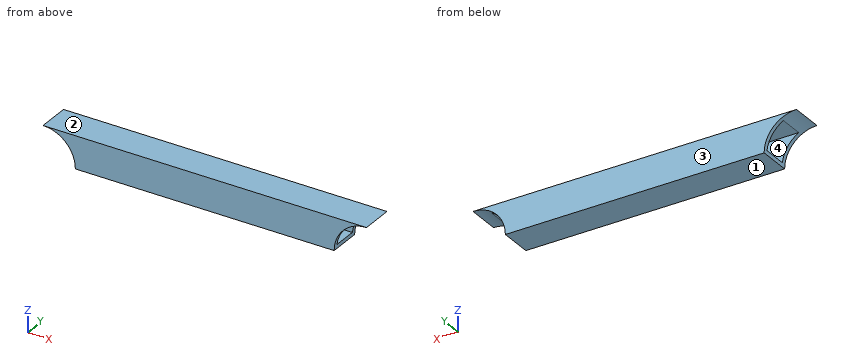
from build123d import *

# Parameters (mm, degrees)
BOSS_EXTRUDE1_DEPTH     = 25.4
CUT_EXTRUDE1_DEPTH      = 163.851117067
CUT_EXTRUDE1_DEPTH_BACK = 163.851117067
SKETCH2_W               = 19.05
SKETCH2_H               = 19.05


with BuildPart() as part:
    # Sketch1 → Boss-Extrude1 (new body)
    with BuildSketch(Plane(origin=(0, 0, 0), x_dir=(1, 0, 0), z_dir=(0, 1, 0))):
        with BuildLine():
            Line((-127, -98.723484187), (127, -98.723484187))
            ThreePointArc((127, -98.723484187), (109.039487758, -91.283996429), (101.6, -73.323484187))
            Line((101.6, -73.323484187), (-101.6, -73.323484187))
            ThreePointArc((-101.6, -73.323484187), (-109.039487758, -91.283996429), (-127, -98.723484187))
        make_face()
    extrude(amount=BOSS_EXTRUDE1_DEPTH)

    # Sketch2 → Cut-Extrude1 (cut, two sides: drawn at the far end of the back side and taken through both)
    with BuildSketch(Plane(origin=(0, 0, 0), x_dir=(0, 0, -1), z_dir=(1, 0, 0)).offset(-CUT_EXTRUDE1_DEPTH_BACK)):
        with Locations((-86.023484187, 12.7)):
            Rectangle(SKETCH2_W, SKETCH2_H)
    extrude(amount=CUT_EXTRUDE1_DEPTH + CUT_EXTRUDE1_DEPTH_BACK, mode=Mode.SUBTRACT)


solid = part.part
Model file for the job. Use its own axes, mm. Face numbers are marked on the shaded views. Round coordinates to 2 decimals unless told otherwise and drop trailing zeros. Order: outer loops, then holes, each group sorted by start corner. A loop starts at its lowest first (then second) coordinate and runs counter-clockwise, first axis right, second up.
(1) Drill centre lines: line 1 (Y direction, x = -57, z = 79.5) (3 decimals); line 2 (Z direction, x = 17, y = 13.25); line 3 (Z direction, x = -112, y = 5.5). Where is each one in solid material? Low to high.
(2) Band-saw the part on C-C (z = 83.5). List the corners of the cut face in (x, y) (3 decimals), then the cut area to 3 significant figures.
(3) Band-saw the part on B-B (x = 41). List the corners of the cut face in (y, z) (3 decimals), then the cut area to 3 significant figures.
(4) Band-saw the part on A-A (y = 8.5). List the corners of the cut face in (x, z).
(5) Pull direction Z, two halves, no side cores. Call the marked faces 1, 2, 3 and 4: released by +Z, released by -Z, zero draft, split by the parting line, or undercut.
(6) Pin check, flat tips, straight feed: pin 1 (10 mm diameter, centred on y = 19.5, z = 90, fed in from -X); pin 2 (5 mm diameter, centred on x = -88.5, z = 76.5, fed in from -Y); pin 3 (6 mm diameter, centred on y = 9, z = 86, fed in from -X). Stop position of each tip, or through.
Verdict:
1. line 1: y = 0 to 3.175, 22.225 to 25.4
1. line 2: z = 73.32 to 76.5, 95.55 to 98.72
1. line 3: z = 95.55 to 98.72
2. outline: (-103.728, 0) - (103.728, 0) - (103.728, 3.175) - (-103.728, 3.175) - close; (-103.728, 22.225) - (103.728, 22.225) - (103.728, 25.4) - (-103.728, 25.4) - close
2. area: 1,320 mm2
3. outline: (0, 73.323) - (25.4, 73.323) - (25.4, 98.723) - (0, 98.723) - close; hole (3.175, 76.498) - (22.225, 76.498) - (22.225, 95.548) - (3.175, 95.548) - close
3. area: 282 mm2
4. outline: (-127, 98.72) arc R25.4 cw to (-114.7, 95.55) - (114.7, 95.55) arc R25.4 cw to (127, 98.72) - close; (-101.8, 76.5) arc R25.4 cw to (-101.6, 73.32) - (101.6, 73.32) arc R25.4 cw to (101.8, 76.5) - close
5. face 1: released by -Z
5. face 2: released by +Z
5. face 3: zero draft
5. face 4: undercut
6. pin 1: stops at x = -112.52
6. pin 2: stops at y = 0
6. pin 3: passes through
